Check sheet for the modelled part. Datum: model origin and axes. Units: mm. Face numbers are marked on the shaded views. A direction names the side the tool comes from. Coordinates: 2 decimals unless noted, no trailing zeros. Write each loop counter-clockwise with the first axis right and the second up, starting at its lowest first coordinate (ties: lowest second). Pieces come first, ordered by that corner, then holes. Notation, with made-up numbers: (12.25, 13.5) - (53.25, 13.5) arc R22 ccw to (53.25, 35.5) - close; hole circle Ø3 at (88.5, -38). An arc over 180 degrees is marked (long way). Write each question's results on one line, items separated by ' | '.
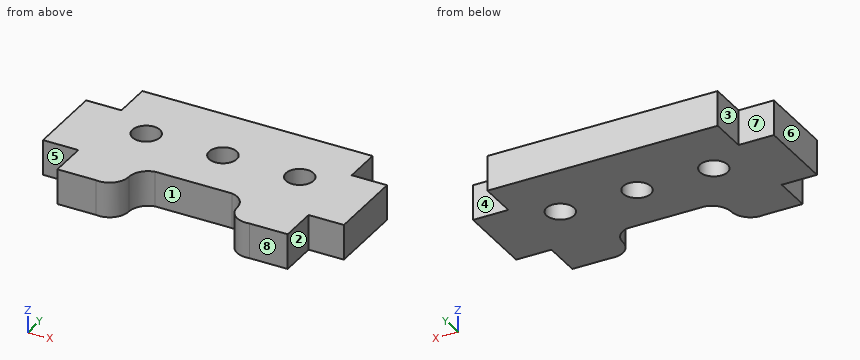
from build123d import *

# Parameters (mm, degrees)
SKETCH1_R           = 2.286
BOSS_EXTRUDE1_DEPTH = 5.842


with BuildPart() as part:
    # Sketch1 → Boss-Extrude1 (new body)
    with BuildSketch(Plane.XY):
        with BuildLine():
            Line((0, 0), (-6.35, 0))
            ThreePointArc((-6.35, 0), (-8.948239117, 0.689575054), (-10.086248608, 3.125))
            ThreePointArc((-10.086248608, 3.125), (-10.825823663, 5.161990509), (-12.7, 6.25))
            Line((-12.7, 6.25), (-25.4, 6.25))
            ThreePointArc((-25.4, 6.25), (-27.274176337, 5.161990509), (-28.013751392, 3.125))
            ThreePointArc((-28.013751392, 3.125), (-29.151760883, 0.689575054), (-31.75, 0))
            Line((-31.75, 0), (-38.1, 0))
            Line((-38.1, 0), (-38.1, 6.25))
            Line((-38.1, 6.25), (-43.942, 6.25))
            Line((-43.942, 6.25), (-43.942, 19.15))
            Line((-43.942, 19.15), (-38.1, 19.15))
            Line((-38.1, 19.15), (-38.1, 25.4))
            Line((-38.1, 25.4), (0, 25.4))
            Line((0, 25.4), (0, 19.15))
            Line((0, 19.15), (5.842, 19.15))
            Line((5.842, 19.15), (5.842, 6.25))
            Line((5.842, 6.25), (0, 6.25))
            Line((0, 6.25), (0, 0))
        make_face()
        with Locations((-6.35, 15.08125)):
            Circle(SKETCH1_R, mode=Mode.SUBTRACT)
        with Locations((-19.05, 15.08125)):
            Circle(SKETCH1_R, mode=Mode.SUBTRACT)
        with Locations((-31.75, 15.08125)):
            Circle(SKETCH1_R, mode=Mode.SUBTRACT)
    extrude(amount=BOSS_EXTRUDE1_DEPTH)


solid = part.part
1. Draft check along X on the marked faces 1, 2 and 3. Enter one of: pulls with the +X half, pulls with the -X half, needs draft (parallel to the pull), parting line crosses it, or undercut.
Values follow:
face 1: undercut | face 2: pulls with the +X half | face 3: pulls with the -X half
2. Sectioned sample at A-A (y = 13.25). Record the cut outline in (x, z).
Values follow:
outline: (-43.94, 0) - (-33.12, 0) - (-33.12, 5.84) - (-43.94, 5.84) - close; (-30.38, 0) - (-20.42, 0) - (-20.42, 5.84) - (-30.38, 5.84) - close; (-17.68, 0) - (-7.72, 0) - (-7.72, 5.84) - (-17.68, 5.84) - close; (-4.98, 0) - (5.84, 0) - (5.84, 5.84) - (-4.98, 5.84) - close
3. Sectioned sample at D-D (y = 2). Record the cut outline in (x, z), then the cut area to 3 significant figures.
Values follow:
outline: (-38.1, 0) - (-28.22, 0) - (-28.22, 5.84) - (-38.1, 5.84) - close; (-9.88, 0) - (0, 0) - (0, 5.84) - (-9.88, 5.84) - close | area: 115 mm^2
4. Access from +Z, -Z, +X, -X, +Y, -Y to the whole of each face (thin tool, end or side, straight path). Record for the marked faces 4, 5, 6, 7 and 8.
Values follow:
face 4: +Z, -Z, +X, +Y | face 5: +Z, -Z, -X, -Y | face 6: +Z, -Z, -X, +Y, -Y | face 7: +Z, -Z, -X, +Y | face 8: +Z, -Z, +X, -Y
5. Sectioned sample at B-B (x = -19.05). Record the cut outline in (y, z).
Values follow:
outline: (6.25, 0) - (12.8, 0) - (12.8, 5.84) - (6.25, 5.84) - close; (17.37, 0) - (25.4, 0) - (25.4, 5.84) - (17.37, 5.84) - close
6. Material ranges on L1, parallel to X at y = 15.25, z = 4.6; L2, parallel to Y at x = -31.75, z = 2.7; L3, parallel to X at y = 13.75, z = 2.8, recorded low to high. Write a range as [from, to].
Values follow:
L1: x = [-43.94, -34.03], [-29.47, -21.33], [-16.77, -8.63], [-4.07, 5.84] | L2: y = [0, 12.8], [17.37, 25.4] | L3: x = [-43.94, -33.61], [-29.89, -20.91], [-17.19, -8.21], [-4.49, 5.84]
7. Sectioned sample at C-C (z = 3.65). Record the cut outline in (x, y) (3 decimals).
Values follow:
outline: (-43.942, 6.25) - (-38.1, 6.25) - (-38.1, 0) - (-31.75, 0) arc R3.175 ccw to (-28.014, 3.125) arc R3.175 cw to (-25.4, 6.25) - (-12.7, 6.25) arc R3.175 cw to (-10.086, 3.125) arc R3.175 ccw to (-6.35, 0) - (0, 0) - (0, 6.25) - (5.842, 6.25) - (5.842, 19.15) - (0, 19.15) - (0, 25.4) - (-38.1, 25.4) - (-38.1, 19.15) - (-43.942, 19.15) - close; hole circle Ø4.572 at (-31.75, 15.081); hole circle Ø4.572 at (-19.05, 15.081); hole circle Ø4.572 at (-6.35, 15.081)
8. Go/stop test with flat-tipped pins: pin 1 (1.8 mm diameter, centred on x = -39.5, z = 3, fed in from -Y); pin 2 (1.8 mm diameter, centred on x = -4, z = 3.5, fed in from -Y); pin 3 (1.5 mm diameter, centred on x = -13, z = 5, fed in from -Y). Record where each tip stops, or that it passes through.
Values follow:
pin 1: stops at y = 6.25 | pin 2: stops at y = 0 | pin 3: stops at y = 6.13
